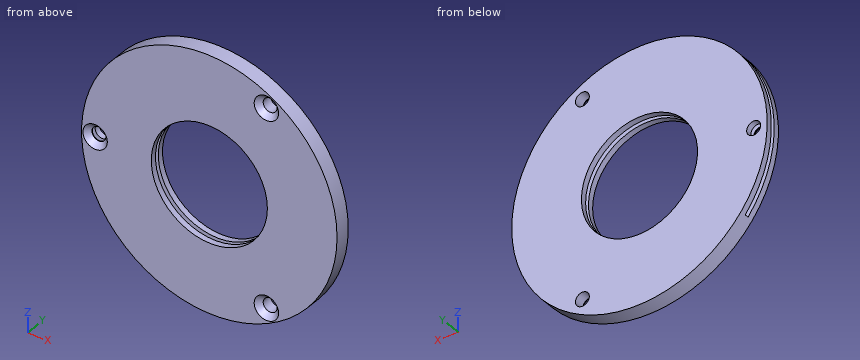
from build123d import *

# Parameters (mm, degrees)
SKETCH1_R                                       = 33
SKETCH1_R_2                                     = 1.5
BOSS_EXTRUDE1_DEPTH                             = 4
CSK_FOR_M3_FLAT_HEAD_MACHINE_SCREW1_D           = 3.6
CSK_FOR_M3_FLAT_HEAD_MACHINE_SCREW1_CSINK_D     = 6.3
CSK_FOR_M3_FLAT_HEAD_MACHINE_SCREW1_CSINK_ANGLE = 90
CORTAR_EXTRUIR1_REACH                           = 6
CROQUIS1_R                                      = 15
CROQUIS2_W                                      = 40
CROQUIS2_H                                      = 1
CORTAR_EXTRUIR2_DEPTH                           = 50


with BuildPart() as part:
    # Sketch1 → Boss-Extrude1 (new body)
    with BuildSketch(Plane(origin=(0, 0, 0), x_dir=(1, 0, 0), z_dir=(0, 1, 0))):
        Circle(SKETCH1_R)
        with Locations((-29.5, 0)):
            Circle(SKETCH1_R_2, mode=Mode.SUBTRACT)
        with Locations((14.75, 25.547749412)):
            Circle(SKETCH1_R_2, mode=Mode.SUBTRACT)
        with Locations((14.75, -25.547749412)):
            Circle(SKETCH1_R_2, mode=Mode.SUBTRACT)
    extrude(amount=BOSS_EXTRUDE1_DEPTH)

    # CSK for M3 Flat Head Machine Screw1 (through all)
    with Locations(Plane(origin=(0, 0, 0), x_dir=(-1, 0, 0), z_dir=(0, -1, 0))):
        with Locations((-14.75, -25.547749412), (29.5, 0), (-14.75, 25.547749412)):
            CounterSinkHole(CSK_FOR_M3_FLAT_HEAD_MACHINE_SCREW1_D / 2, CSK_FOR_M3_FLAT_HEAD_MACHINE_SCREW1_CSINK_D / 2, counter_sink_angle=CSK_FOR_M3_FLAT_HEAD_MACHINE_SCREW1_CSINK_ANGLE)

    # Croquis1 → Cortar-Extruir1 (cut, up to next)
    with BuildSketch(Plane.XZ, mode=Mode.PRIVATE) as cortar_extruir1_sk1:
        Circle(CROQUIS1_R)
    cortar_extruir1_tool1 = extrude(cortar_extruir1_sk1.sketch, amount=-CORTAR_EXTRUIR1_REACH, mode=Mode.PRIVATE) & part.part
    add(cortar_extruir1_tool1.solids().sort_by_distance((0, 0, 0))[0], mode=Mode.SUBTRACT)

    # Croquis2 → Cortar-Extruir2 (cut)
    with BuildSketch(Plane.ZY.offset(33)):
        with Locations((0, 2)):
            Rectangle(CROQUIS2_W, CROQUIS2_H)
    extrude(amount=-CORTAR_EXTRUIR2_DEPTH, mode=Mode.SUBTRACT)


solid = part.part
Model file for the job. Use its own axes, mm. Give positions to 0.01 mm unless a question says otherwise; leave off trailing zeros. Write each loop counter-clockwise with the first axis right and the second up, starting at its lowest first coordinate (ties: lowest second). Pieces come first, ordered by that corner, then holes. Notation, with made-up numbers: M 28,76.5 L 74,76.5 A18 cw 74,103.5 Z; hole C 45,-3.5 d4. An arc over 180 degrees is marked long. One line per item, written item: value. Start each with the question number.
Q1. Probe probe 1 along Y at (x, z) = (15, 7); probe 2 along Z at (x, y) = (0, 1.05); probe 3 along X at (y, z) = (0.9, 8.5). List the from-to ranges inside material, lowest first. Write a range as [from, to].
Q2. Saw through at B-B, the plane z = 0. Write the cut outline in (x, y).
Q3. Saw through at C-C, the plane x = -29.5. Write the cut outline in (y, z).
Q4. Saw through at D-D, the plane z = 10. Write the cut outline in (x, y), plus the area to 3 significant figures.
Q5. Saw through at A-A, the plane x = 0. Write the cut outline in (y, z), plus the area to 3 significant figures.
Q6. Drop flat-ended pins along their axis: pin 1 Ø4.5 at (x, z) = (14.75, -25.55) entering from -Y; pin 2 Ø1 at (y, z) = (1.5, -16.5) entering from +X; pin 3 Ø6 at (x, z) = (-29.5, 0) entering from -Y. Give the stop position or say it passes through.
Output values:
1. probe 1: y = [0, 1.5], [2.5, 4]
1. probe 2: z = [-33, -15], [15, 33]
1. probe 3: x = [-31.89, -12.36], [12.36, 31.89]
2. outline: M -33,0 L -32.65,0 L -31.3,1.35 L -31.3,1.5 L -33,1.5 Z; M -33,2.5 L -31.3,2.5 L -31.3,4 L -33,4 Z; M -27.7,1.35 L -26.35,0 L -15,0 L -15,1.5 L -27.7,1.5 Z; M -27.7,2.5 L -15,2.5 L -15,4 L -27.7,4 Z; M 15,0 L 33,0 L 33,4 L 15,4 L 15,2.5 L 17,2.5 L 17,1.5 L 15,1.5 Z
3. outline: M 0,-14.79 L 1.5,-14.79 L 1.5,-1.8 L 1.35,-1.8 L 0,-3.15 Z; M 0,3.15 L 1.35,1.8 L 1.5,1.8 L 1.5,14.79 L 0,14.79 Z; M 2.5,-14.79 L 4,-14.79 L 4,-1.8 L 2.5,-1.8 Z; M 2.5,1.8 L 4,1.8 L 4,14.79 L 2.5,14.79 Z
4. outline: M -31.45,0 L -11.18,0 L -11.18,1.5 L -31.45,1.5 Z; M -31.45,2.5 L -11.18,2.5 L -11.18,4 L -31.45,4 Z; M 11.18,0 L 31.45,0 L 31.45,4 L 11.18,4 L 11.18,2.5 L 17,2.5 L 17,1.5 L 11.18,1.5 Z
4. area: 136 mm²
5. outline: M 0,-33 L 4,-33 L 4,-15 L 2.5,-15 L 2.5,-20 L 1.5,-20 L 1.5,-15 L 0,-15 Z; M 0,15 L 1.5,15 L 1.5,20 L 2.5,20 L 2.5,15 L 4,15 L 4,33 L 0,33 Z
5. area: 134 mm²
6. pin 1: stops at y = 0.9
6. pin 2: stops at x = 28.86
6. pin 3: stops at y = 0.15
